Could you check a few things on this model? Use its own coordinates, in mm. A direction names the side the tool comes from. Give positions to 0.01 mm unless a question says otherwise; leave off trailing zeros. Loops run counter-clockwise (first coordinate to the right, second up) from the corner with the lowest first, then second, coordinate; pieces in that order, holes last. Notation, with made-up numbers: M 73.25,83 L 92.25,83 A20 cw 92.25,121 Z; hole C 72.5,10.5 d1. An arc over 180 degrees is marked long. Answer in a Markdown table with one row per item. Add a question column.
1. Thinking about a two-plate mould opening in Z: for faces 4 (the flat face through (-4, 3, -30)), 5 (the flat face through (-7, 0.4, -30)), 6 (the cylindrical face through (-7.5, 2.4, -32.2)), which applies, released by +Z, released by -Z, zero draft, split by the parting line, or undercut?
2. I'm going to push flat-ended pins straight in: pin 1 Ø3 at (x, z) = (-8, 2) entering from -Y; pin 2 Ø3.5 at (y, z) = (2, 3) entering from +X; pin 3 Ø0.6 at (x, y) = (-7.5, 1) entering from +Z. Where does each tip first touch, or does it pass through?
3. If we section it at C-C on y = 2.5: List the corners of the cut face in (x, z) for me.
4. I need wall thicknesses on line 1 along X through (y, z) = (0.55, -7); line 2 along Z through (x, y) = (-7, 0.75); line 3 along Z through (x, y) = (-5.5, 3). Which ranges of each line are inside material? Lowest first, please. Write a range as from..to.
5. If we section it at D-D on z = -12.5: List the corners of the cut face in (x, y) for me.
6. If we section it at B-B on z = -7: List the corners of the cut face in (x, y) for me.
7. If we section it at A-A on x = -7: List the corners of the cut face in (y, z) for me, then the cut area to 3 significant figures.
8. Which directions (+Z, -Z, +X, -X, +Y, -Y) give clear straight access to the entire face, cutting with the end or side of a thin tool? Please do faces 1 (the flat face through (-7, 4, 2)), 2 (the flat face through (-10, 3, -30)), 3 (the flat face through (-12.5, 0.5, -30)).
Autodesk Inventor part; units mm, degrees
ref_plane "YZ Plane" through (0, 0, 0) normal (1, 0, 0) x (0, 1, 0)
ref_plane "XZ Plane" through (0, 0, 0) normal (0, 1, 0) x (-1, 0, 0)
ref_plane "XY Plane" through (0, 0, 0) normal (0, 0, 1) x (1, 0, 0)
sketch "Sketch1" plane through (0, 0, 0) normal (0, 1, 0) x (-1, 0, 0)
  line L0 (0, 0) -> (14, 0)
  line L1 (14, 0) -> (14, -30)
  line L2 (14, -30) -> (0, -30)
  line L3 (0, -30) -> (0, 0)
  dimension "d0" = 14
  dimension "d1" = 30
extrude "Extrusion1" add sketch "Sketch1" along normal blind 1
sketch "Sketch2" plane through (0, 0, -30) normal (0, 0, -1) x (-1, 0, 0)
  circle A0 centre (4, 2.5) radius 2.5
  circle A1 centre (10, 2.5) radius 2.5
  line L0 (0, 0) -> (14, 0)
  line L1 (14, 0) -> (14, 1)
  line L2 (0, 0) -> (0, 1)
  point P0 (14, 0.5)
  point P1 (0, 0.5)
  dimension "d4" = 5
  dimension "d5" = 5
  dimension "d6" = 2.5
  dimension "d7" = 4
  dimension "d8" = 4
extrude "Extrusion2" add sketch "Sketch2" along normal blind 7
fillet "Fillet1" radius 2.5 2 edges at (-1.5, 2.5, -37) (-7.5, 2.5, -37)
sketch "Sketch3" plane through (0, 1, 0) normal (0, 1, 0) x (1, 0, 0)
  line L0 (-10, 0.5) -> (-4, 0.5)
  line L1 (-4, 0.5) -> (-4, 3)
  line L2 (-4, 3) -> (-10, 3)
  line L3 (-10, 3) -> (-10, 0.5)
  line L4 (0, 0) -> (0, 30)
  line L5 (-14, 0) -> (0, 0)
  point P0 (-7, 0.5)
  dimension "d12" = 6
  dimension "d13" = 4
  dimension "d14" = 2.5
  dimension "d15" = 0.5
extrude "Extrusion3" add sketch "Sketch3" along normal blind 3
sketch "Sketch4" plane through (-10, 1, -0.5) normal (0, 0, 1) x (1, 0, 0)
  line L0 (6, 3) -> (0, 3)
  line L1 (6, 0) -> (6, 3)
  line L2 (0, 3) -> (6, 3)
  line L3 (6, 3) -> (6, 0.5)
  line L4 (6, 0.5) -> (0, 0.5)
  line L5 (0, 0.5) -> (0, 3)
  point P0 (10, -1)
  dimension "d18" = 2.5
extrude "Extrusion4" add sketch "Sketch4" along normal blind 7
sketch "Sketch5" plane through (0, 1, 0) normal (0, 1, 0) x (1, 0, 0)
  line L0 (-2, 18) -> (-8, 18)
  line L1 (-8, 18) -> (-8, 12)
  line L2 (-8, 12) -> (-2, 12)
  line L3 (-2, 12) -> (-2, 18)
  line L4 (0, 0) -> (0, 30)
  line L5 (-1.5, 30) -> (-6.5, 30)
  point P0 (-2, 15)
  point P1 (-6, 30)
  point P2 (-2, 30)
  dimension "d21" = 6
  dimension "d22" = 6
  dimension "d23" = 2
  dimension "d24" = 12
extrude "Extrusion5" add sketch "Sketch5" along normal blind 5
sketch "Sketch6" plane through (0, 1, 0) normal (0, 1, 0) x (1, 0, 0)
  circle A0 centre (-7, 7) radius 1.5
  line L0 (-14, 0) -> (0, 0)
  line L1 (0, 0) -> (0, 30)
  dimension "d27" = 3
  dimension "d28" = 7
  dimension "d29" = 7
extrude "Extrusion6" cut sketch "Sketch6" against normal through all
properties part number "IR"
Results:
| question | item | result |
|---|---|---|
| 1 | face 4 | undercut |
| 1 | face 5 | released by -Z |
| 1 | face 6 | zero draft |
| 2 | pin 1 | y = 1.5 |
| 2 | pin 2 | x = -4 |
| 2 | pin 3 | z = 0 |
| 3 | outline | M -12.5,-34.5 A2.5 ccw -7.5,-34.5 L -7.5,-30 L -12.5,-30 Z; M -10,-3 L -4,-3 L -4,6.5 L -10,6.5 Z; M -8,-18 L -2,-18 L -2,-12 L -8,-12 Z; M -6.5,-34.5 A2.5 ccw -1.5,-34.5 L -1.5,-30 L -6.5,-30 Z |
| 4 | line 1 | -14..-8.5, -5.5..0 |
| 4 | line 2 | -30..-8.5, -5.5..0 |
| 4 | line 3 | -36.44..-30, -18..-12, -3..6.5 |
| 5 | outline | M -14,0 L 0,0 L 0,1 L -2,1 L -2,6 L -8,6 L -8,1 L -14,1 Z |
| 6 | outline | M -14,0 L -8.5,0 L -8.5,1 L -14,1 Z; M -5.5,0 L 0,0 L 0,1 L -5.5,1 Z |
| 7 | outline | M 0,-30 L 1,-30 L 1,-18 L 6,-18 L 6,-12 L 1,-12 L 1,-8.5 L 0,-8.5 Z; M 0,-5.5 L 1,-5.5 L 1,-3 L 4,-3 L 4,6.5 L 1.5,6.5 L 1.5,-0.5 L 1,-0.5 L 1,0 L 0,0 Z |
| 7 | area | 82.0 mm2 |
| 8 | face 1 | +Z, +X, -X, +Y |
| 8 | face 2 | +X, -X, +Y |
| 8 | face 3 | -Z, -X, -Y |
